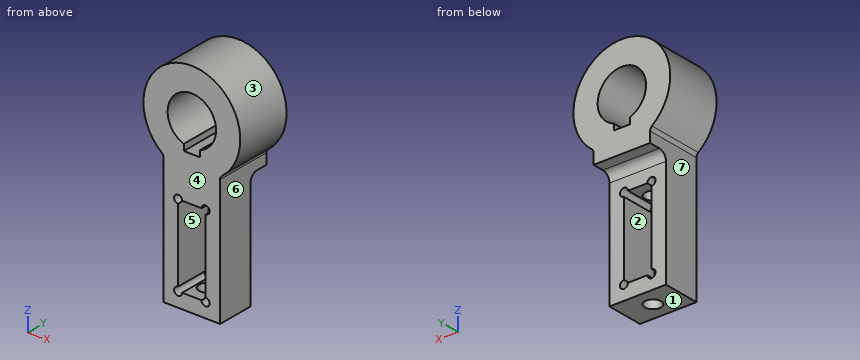
from build123d import *

# Parameters (mm, degrees)
BOSS_EXTRUDE1_DEPTH = 35
SKETCH2_W           = 35
SKETCH2_H           = 12
CUT_EXTRUDE1_DEPTH  = 72
FILLET1_R           = 5
FILLET2_R           = 3
SKETCH3_R           = 5
CUT_EXTRUDE2_DEPTH  = 65


with BuildPart() as part:
    # Sketch1 → Boss-Extrude1 (new body)
    with BuildSketch(Plane(origin=(0, 0, 0), x_dir=(1, 0, 0), z_dir=(0, 1, 0))):
        with BuildLine():
            Line((-17.5, 104.366985862), (17.5, 104.366985862))
            Line((17.5, 104.366985862), (17.5, 24.366985862))
            ThreePointArc((17.5, 24.366985862), (0, -30), (-17.5, 24.366985862))
            Line((-17.5, 24.366985862), (-17.5, 104.366985862))
        make_face()
        with BuildLine():
            Line((-6, 95.366985862), (6, 95.366985862))
            ThreePointArc((6, 95.366985862), (10.267766953, 97.134752815), (8.5, 92.866985862))
            Line((8.5, 92.866985862), (8.5, 47.866985862))
            ThreePointArc((8.5, 47.866985862), (10.267766953, 43.599218909), (6, 45.366985862))
            Line((6, 45.366985862), (-6, 45.366985862))
            ThreePointArc((-6, 45.366985862), (-10.267766953, 43.599218909), (-8.5, 47.866985862))
            Line((-8.5, 47.866985862), (-8.5, 92.866985862))
            ThreePointArc((-8.5, 92.866985862), (-10.267766953, 97.134752815), (-6, 95.366985862))
        make_face(mode=Mode.SUBTRACT)
        with BuildLine():
            Line((5, 18), (5, 14.142135624))
            ThreePointArc((5, 14.142135624), (0, -15), (-5, 14.142135624))
            Line((-5, 14.142135624), (-5, 18))
            Line((-5, 18), (5, 18))
        make_face(mode=Mode.SUBTRACT)
    extrude(amount=BOSS_EXTRUDE1_DEPTH)

    # Sketch2 → Cut-Extrude1 (cut)
    with BuildSketch(Plane(origin=(0, 0, -104.366985862), x_dir=(-1, 0, 0), z_dir=(0, 0, -1))):
        with Locations((0, 29)):
            Rectangle(SKETCH2_W, SKETCH2_H)
    extrude(amount=-CUT_EXTRUDE1_DEPTH, mode=Mode.SUBTRACT)

    # Fillet1
    fillet1_edges = [part.edges().sort_by_distance(p)[0] for p in [
        (0, 23, -32.366985862),
    ]]
    fillet(fillet1_edges, radius=FILLET1_R)

    # Fillet2
    fillet2_edges = [part.edges().sort_by_distance(p)[0] for p in [
        (-17.5, 17.5, -24.366985862),
        (17.5, 17.5, -24.366985862),
    ]]
    fillet(fillet2_edges, radius=FILLET2_R)

    # Sketch3 → Cut-Extrude2 (cut)
    with BuildSketch(Plane(origin=(0, 0, -104.366985862), x_dir=(-1, 0, 0), z_dir=(0, 0, -1))):
        with Locations((0, 11.5)):
            Circle(SKETCH3_R)
    extrude(amount=-CUT_EXTRUDE2_DEPTH, mode=Mode.SUBTRACT)


solid = part.part
Geometry check sheet. Reference: the model listing, model coordinates, mm. Face numbers are marked on the shaded views. A direction names the side the tool comes from. Give positions to 0.01 mm unless a question says otherwise; leave off trailing zeros. Order: outer loops, then holes, each group sorted by start corner. A loop starts at its lowest first (then second) coordinate and runs counter-clockwise, first axis right, second up. Notation, with made-up numbers: M 19,-27.75 L 75,-27.75 A28 ccw 75,-6.75 Z; hole C 54,-24 d5. An arc over 180 degrees is marked long. Use a Markdown table: item, result.
Item 1: Section check D-D (y = 30). Record the cut outline in (x, z), and give its area (3 significant figures).
Answers follow:
| item | result |
|---|---|
| outline | M -18.64,-23.51 A3 cw -17.5,-25.86 L -17.5,-32.37 L 17.5,-32.37 L 17.5,-25.86 A3 cw 18.64,-23.51 A30 ccw long Z; hole M -5,-18 L 5,-18 L 5,-14.14 A15 ccw long -5,-14.14 Z |
| area | 2,230 mm2 |
Item 2: Depth check by flat-ended pin: P1, Ø13, axis at x = 0, y = 11.5, coming from the +Z side; P2, Ø4, axis at y = 14.5, z = -72.5, coming from the -X side; P3, Ø3, axis at y = 26, z = -15.5, coming from the +X side. Enter the tip coordinate at first touch or a pass-through.
Answers follow:
| item | result |
|---|---|
| P1 | stops at z = 30 |
| P2 | stops at x = -17.5 |
| P3 | stops at x = 26.53 |
Item 3: Section check C-C (y = 4.5). Record the cut outline in (x, z).
Answers follow:
| item | result |
|---|---|
| outline | M -18.64,-23.51 A3 cw -17.5,-25.86 L -17.5,-104.37 L 17.5,-104.37 L 17.5,-25.86 A3 cw 18.64,-23.51 A30 ccw long Z; hole M -8.5,-92.87 A2.5 ccw long -6,-95.37 L 6,-95.37 A2.5 ccw long 8.5,-92.87 L 8.5,-47.87 A2.5 ccw long 6,-45.37 L -6,-45.37 A2.5 ccw long -8.5,-47.87 Z; hole M -5,-18 L 5,-18 L 5,-14.14 A15 ccw long -5,-14.14 Z |
Item 4: Section check B-B (x = 0). Record the cut outline in (y, z).
Answers follow:
| item | result |
|---|---|
| outline | M 0,-104.37 L 6.5,-104.37 L 6.5,-95.37 L 0,-95.37 Z; M 0,-45.37 L 6.5,-45.37 L 6.5,-39.37 L 16.5,-39.37 L 16.5,-45.37 L 23,-45.37 L 23,-37.37 A5 cw 28,-32.37 L 35,-32.37 L 35,-18 L 0,-18 Z; M 0,15 L 35,15 L 35,30 L 0,30 Z; M 16.5,-104.37 L 23,-104.37 L 23,-95.37 L 16.5,-95.37 Z |
Item 5: Section check A-A (z = -56.5). Record the cut outline in (x, y).
Answers follow:
| item | result |
|---|---|
| outline | M -17.5,0 L -8.5,0 L -8.5,23 L -17.5,23 Z; M 8.5,0 L 17.5,0 L 17.5,23 L 8.5,23 Z |
Item 6: Material ranges on line 1 along Z through (x, y) = (9, 15.5); line 2 along Z through (x, y) = (0, 33); line 3 along Z through (x, y) = (13, 25.5), recorded low to high.
Answers follow:
| item | result |
|---|---|
| line 1 | z = -104.37 to -97.82, -92.92 to -47.82, -42.92 to -12, 12 to 28.62 |
| line 2 | z = -32.37 to -18, 15 to 30 |
| line 3 | z = -33.04 to -7.48, 7.48 to 27.04 |
Item 7: Draft check along Z on the marked faces 1, 2, 3 and 4. Enter one of: +Z half, -Z half, draft (parallel to the pull), parting line (faces both ways), or undercut.
Answers follow:
| item | result |
|---|---|
| face 1 | -Z half |
| face 2 | undercut |
| face 3 | parting line |
| face 4 | draft |
Item 8: Tool access check on the marked faces 5, 6 and 7. Record the directions out of +Z, -Z, +X, -X, +Y, -Y that give a thin tool (end or side, any length) a straight path to the whole face; none if there is none.
Answers follow:
| item | result |
|---|---|
| face 5 | +Y, -Y |
| face 6 | -Z, +X, +Y, -Y |
| face 7 | -Z, -X, +Y, -Y |
